from build123d import *

# Parameters (mm, degrees)
SKETCH1_W           = 47.09
SKETCH1_H           = 10
BOSS_EXTRUDE1_DEPTH = 2


with BuildPart() as part:
    # Sketch1 → Boss-Extrude1 (new body)
    with BuildSketch(Plane(origin=(0, 0, 0), x_dir=(1, 0, 0), z_dir=(0, 1, 0))):
        with Locations((-13.079545455, 1.78030303)):
            Rectangle(SKETCH1_W, SKETCH1_H)
        with BuildLine():
            add(Edge.make_bspline(
                [(-9.754545455, 1.78030303), (-9.754545455, 1.044100491), (-8.642482329, -0.428304587), (-4.704545455, -1.315393161), (-0.76660858, -0.428304587), (0.901486108, 1.78030303), (-0.76660858, 3.988910648), (-4.704545455, 4.875999221), (-8.642482329, 3.988910648), (-9.754545455, 2.51650557), (-9.754545455, 1.78030303)],
                knots=[0, 0, 0, 0, 0.785398163, 1.570796327, 2.35619449, 3.141592654, 3.926990817, 4.71238898, 5.497787144, 6.283185307, 6.283185307, 6.283185307, 6.283185307], degree=3))
        make_face(mode=Mode.SUBTRACT)
        with BuildLine():
            add(Edge.make_bspline(
                [(-16.404545455, 1.78030303), (-16.404545455, 1.044100491), (-17.51660858, -0.428304587), (-21.454545455, -1.315393161), (-25.392482329, -0.428304587), (-27.060577017, 1.78030303), (-25.392482329, 3.988910648), (-21.454545455, 4.875999221), (-17.51660858, 3.988910648), (-16.404545455, 2.51650557), (-16.404545455, 1.78030303)],
                knots=[0, 0, 0, 0, 0.785398163, 1.570796327, 2.35619449, 3.141592654, 3.926990817, 4.71238898, 5.497787144, 6.283185307, 6.283185307, 6.283185307, 6.283185307], degree=3))
        make_face(mode=Mode.SUBTRACT)
    extrude(amount=BOSS_EXTRUDE1_DEPTH)


solid = part.part
Can you work these out from the model? Positions are in its coordinate system, mm. Round coordinates to 2 decimals unless told otherwise and drop trailing zeros. Write each question's results on one line, items separated by ' | '. Start each with the question number.
Item 1: Thinking about a two-plate mould opening in Z: for faces 1 (the flat face through (-13, 1, -6.78)), 2 (the flat face through (-13, 2, -2)), 3 (the flat face through (-13, 1, 3.22)), which applies, +Z half, -Z half, draft (parallel to the pull), parting line (faces both ways), or undercut?
Item 2: If we section it at A-A, the plane z = -2.75: State how many separate pieces and enclosed holes the cut face has, then the cut area to 3 significant figures.
Item 3: Please list where these lines run through material, in increasing order: L1, parallel to Z at x = -5, y = 0.4; L2, parallel to X at y = 1.4, z = -0.75; L3, parallel to X at y = 0.75, z = -1.5.
Results:
1) face 1: -Z half | face 2: draft | face 3: +Z half
2) separate pieces: 3 | enclosed holes: 0 | area: 56.3 mm2
3) L1: z = -6.78 to -4.58, 1.01 to 3.22 | L2: x = -36.62 to -26.14, -16.77 to -9.39, -0.02 to 10.47 | L3: x = -36.62 to -26.48, -16.43 to -9.73, 0.32 to 10.47
